CAD build for the part. Positions are in the model's coordinates, mm. Round coordinates to 2 decimals unless told otherwise and drop trailing zeros. Order: outer loops, then holes, each group sorted by start corner. A loop starts at its lowest first (then second) coordinate and runs counter-clockwise, first axis right, second up. Notation, with made-up numbers: M -0.75,-40 L 26.25,-40 A24 ccw 26.25,-25 Z; hole C 65.5,8 d7. An arc over 180 degrees is marked long. Answer as a JSON object with one key per item and string values. Group by question number.
```python
from build123d import *

# Parameters (mm, degrees)
SKETCH1_R           = 3
SKETCH1_R_2         = 2.5
SKETCH1_R_3         = 2.75
BOSS_EXTRUDE1_DEPTH = 5


with BuildPart() as part:
    # Sketch1 → Boss-Extrude1 (new body)
    with BuildSketch(Plane.XY):
        with BuildLine():
            Line((30.000692042, 92.545526446), (235.000692042, 92.545526446))
            ThreePointArc((235.000692042, 92.545526446), (238.536225947, 91.081060352), (240.000692042, 87.545526446))
            Line((240.000692042, 87.545526446), (240.000692042, -52.454473554))
            ThreePointArc((240.000692042, -52.454473554), (238.536225947, -55.99000746), (235.000692042, -57.454473554))
            Line((235.000692042, -57.454473554), (30.000692042, -57.454473554))
            ThreePointArc((30.000692042, -57.454473554), (-44.999307958, 17.545526446), (30.000692042, 92.545526446))
        make_face()
        with Locations((184.000692042, 60.045526446)):
            Circle(SKETCH1_R, mode=Mode.SUBTRACT)
        with Locations((184.000692042, -24.954473554)):
            Circle(SKETCH1_R, mode=Mode.SUBTRACT)
        with Locations((34.000692042, 60.045526446)):
            Circle(SKETCH1_R, mode=Mode.SUBTRACT)
        with Locations((34.000692042, -24.954473554)):
            Circle(SKETCH1_R, mode=Mode.SUBTRACT)
        with Locations((-34.999307958, 17.545526446)):
            Circle(SKETCH1_R_2, mode=Mode.SUBTRACT)
        with Locations((30.000692042, 36.045526446)):
            Circle(SKETCH1_R_3, mode=Mode.SUBTRACT)
        with Locations((30.000692042, -0.954473554)):
            Circle(SKETCH1_R_3, mode=Mode.SUBTRACT)
        with Locations((30.000692042, -47.454473554)):
            Circle(SKETCH1_R_2, mode=Mode.SUBTRACT)
        with Locations((30.000692042, 82.545526446)):
            Circle(SKETCH1_R_2, mode=Mode.SUBTRACT)
        with Locations((230.000692042, -47.454473554)):
            Circle(SKETCH1_R_2, mode=Mode.SUBTRACT)
        with Locations((230.000692042, 82.545526446)):
            Circle(SKETCH1_R_2, mode=Mode.SUBTRACT)
        with Locations((130.000692042, 82.545526446)):
            Circle(SKETCH1_R_2, mode=Mode.SUBTRACT)
        with Locations((130.000692042, -47.454473554)):
            Circle(SKETCH1_R_2, mode=Mode.SUBTRACT)
    extrude(amount=BOSS_EXTRUDE1_DEPTH)


solid = part.part
```
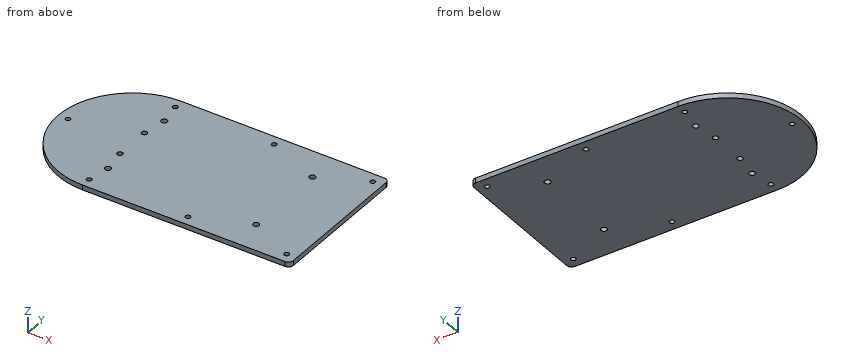
Item 1: Cut at B-B, the plane x = -4. Give the cut face in (y, z), and give its area (3 significant figures).
Item 2: Drill centre lines: line 1 (Y direction, x = 35, z = 3.7); line 2 (X direction, y = 60, z = 1.6); line 3 (X direction, y = 59, z = 4.85). Where is each one in solid material? Low to high. Write a range as [from, to].
Item 3: Cut at A-A, the plane z = 3.05. Give the number of separate pieces and of enclosed holes in the cut face, and give its area (3 significant figures).
Item 4: Cut at C-C, the plane y = 76. Give the cut face in (x, z).
Response values:
{
 "1": {"outline": "M -49.3,0 L 84.4,0 L 84.4,5 L -49.3,5 Z", "area": "669 mm^2"},
 "2": {"line 1": "[-57.45, -27.78], [-22.13, 57.22], [62.87, 92.55]", "line 2": "[-31.83, 31], [37, 181], [187, 240]", "line 3": "[-32.5, 31.19], [36.81, 181.19], [186.81, 240]"},
 "3": {"separate pieces": "1", "enclosed holes": "13", "area": "40,000 mm^2"},
 "4": {"outline": "M -16.99,0 L 240,0 L 240,5 L -16.99,5 Z"}
}
